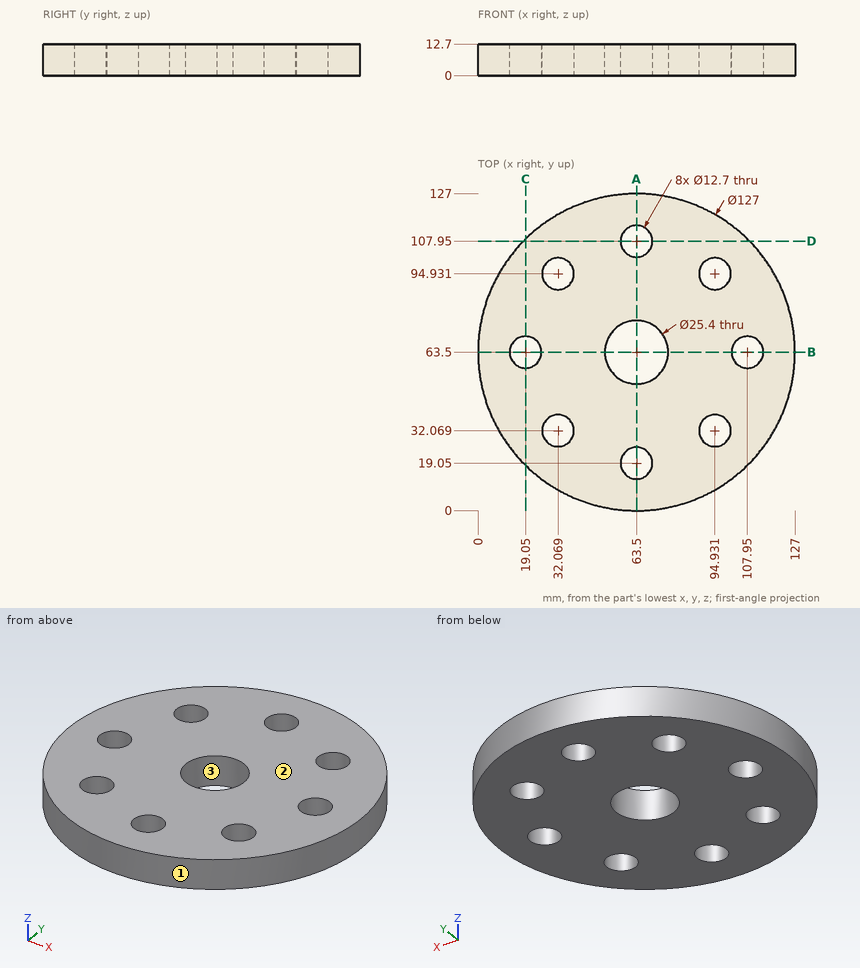
Answer from the drawing. Dimensions are ordinates in mm from the lowest x, y and z of the part. Give positions to 0.01 mm unless a question says otherwise; leave off trailing zeros. Write each loop counter-clockwise with the first axis right and the second up, starting at its lowest first coordinate (ties: lowest second). Pieces come first, ordered by that corner, then holes. Notation, with made-up numbers: (56, 79.25) - (86, 79.25) arc R20 ccw to (86, 100.25) - close; hole circle Ø5 at (-11, 8.25). An arc over 180 degrees is marked (long way). One line per item, written item: value. Start each with the question number.
1. Consider probe 1 along Y at (x, z) = (63.5, 4); probe 2 along Y at (x, z) = (36.5, 10.75); probe 3 along Y at (x, z) = (61.5, 9). Determine where each line is inside the solid, lowest interval first.
2. For a pull along Y with two mould halves and no side action, classify the marked faces 1, 2 and 3 as +Y half, -Y half, draft (parallel to the pull), parting line (faces both ways), or undercut.
3. Given pin 1 (15 mm diameter, centred on x = 63.5, y = 63.5, fed in from +Z); pin 2 (1.5 mm diameter, centred on x = 34.5, z = 10.5, fed in from -Y); pin 3 (1 mm diameter, centred on y = 87.5, z = 8.5, fed in from -X); pin 4 (4 mm diameter, centred on x = 61.5, z = 10, fed in from +Y), each flat-ended and moving along its own axis, determine where each tip first touches the part or whether it passes through.
4. Find section C-C (x = 19.05). Write down the section's boundary in (y, z).
5. Find section A-A (x = 63.5). Write down the section's boundary in (y, z), then the cut area to 3 significant figures.
Geometry results:
1. probe 1: 0 to 12.7, 25.4 to 50.8, 76.2 to 101.6, 114.3 to 127
1. probe 2: 6.03 to 27.52, 36.62 to 90.38, 99.48 to 120.97
1. probe 3: 0.03 to 13.02, 25.08 to 50.96, 76.04 to 101.92, 113.98 to 126.97
2. face 1: parting line
2. face 2: draft
2. face 3: undercut
3. pin 1: through
3. pin 2: y = 6.63
3. pin 3: x = 4.51
3. pin 4: y = 127
4. outline: (18.15, 0) - (57.15, 0) - (57.15, 12.7) - (18.15, 12.7) - close; (69.85, 0) - (108.85, 0) - (108.85, 12.7) - (69.85, 12.7) - close
5. outline: (0, 0) - (12.7, 0) - (12.7, 12.7) - (0, 12.7) - close; (25.4, 0) - (50.8, 0) - (50.8, 12.7) - (25.4, 12.7) - close; (76.2, 0) - (101.6, 0) - (101.6, 12.7) - (76.2, 12.7) - close; (114.3, 0) - (127, 0) - (127, 12.7) - (114.3, 12.7) - close
5. area: 968 mm2
